Could you check a few things on this model? Use its own coordinates, in mm. Give positions to 0.01 mm unless a question says otherwise; leave off trailing zeros. Loops run counter-clockwise (first coordinate to the right, second up) from the corner with the lowest first, then second, coordinate; pieces in that order, holes last. Notation, with made-up numbers: M -34.5,-25.75 L -17.5,-25.75 A35 ccw -17.5,12.25 Z; hole C 4.25,-11 d11. An arc over 180 degrees is marked long. Use a Markdown table: item, result. Add a question column.
1) Suppose I cut it at B-B on y = -25.5. List the corners of the cut face in (x, z) for me, and give its area (3 significant figures).
2) Suppose I cut it at C-C on y = 26.5. List the corners of the cut face in (x, z) for me.
3) If I drill on line 1 along Y through (x, z) = (-42.5, 0.7); line 2 along X through (y, z) = (-60.5, 0.4); line 3 along X through (y, z) = (113, 0.55), over which ranges is the centre line in solid material (lowest first)? Write a range as [from, to].
4) Suppose I cut it at A-A on z = 1.05. Count the separate pieces of the cut face and the enclosed holes in it, and give its area (3 significant figures).
```python
from build123d import *

# Parameters (mm, degrees)
RESSALTO_EXTRUS_O1_DEPTH                     = 1.5
ESCAREADO_PARA_PARAFUSO_ALLEN_SEXTAV_2_COUNT = 2
ESCAREADO_PARA_PARAFUSO_ALLEN_SEXTAV_2_PITCH = 16.970294761
ESCAREADO_PARA_PARAFUSO_ALLEN_SEXTAV_3_COUNT = 2
ESCAREADO_PARA_PARAFUSO_ALLEN_SEXTAV_3_PITCH = 126.454837383
ESCAREADO_PARA_PARAFUSO_ALLEN_SEXTAV_4_COUNT = 2
ESCAREADO_PARA_PARAFUSO_ALLEN_SEXTAV_4_PITCH = 137.976919064
ESCAREADO_PARA_PARAFUSO_ALLEN_SEXTAV_5_COUNT = 2
ESCAREADO_PARA_PARAFUSO_ALLEN_SEXTAV_5_PITCH = 225.316554427
ESCAREADO_PARA_PARAFUSO_ALLEN_SEXTAV_6_COUNT = 2
ESCAREADO_PARA_PARAFUSO_ALLEN_SEXTAV_6_PITCH = 252.205372066
ESCAREADO_PARA_PARAFUSO_ALLEN_SEXTAV_7_COUNT = 2
ESCAREADO_PARA_PARAFUSO_ALLEN_SEXTAV_7_PITCH = 229.941146022
ESCAREADO_PARA_PARAFUSO_ALLEN_SEXTAV_8_COUNT = 2
ESCAREADO_PARA_PARAFUSO_ALLEN_SEXTAV_8_PITCH = 200.082309648


with BuildPart() as part:
    # Esboço1 → Ressalto-extrusão1 (new body)
    with BuildSketch(Plane.XY):
        Polygon((59.050720106, 130.399321825), (-58.939675618, 130.399321825), (-92.944477756, 89.873976712), (-92.944477756, 38.765530101), (-49.944477756, -12.47987438), (-49.944477756, -128.492963544), (-48.624354865, -129.600678175), (48.735399354, -129.600678175), (50.055522244, -128.492963544), (50.055522244, -12.47987438), (93.055522244, 38.765530101), (93.055522244, 89.873976712), align=None)
    extrude(amount=RESSALTO_EXTRUS_O1_DEPTH)

    # Esboço4 → Escareado para parafuso Allen sextavado escareado de M41 (revolve, cut)
    with BuildSketch(Plane(origin=(-63.227418691, 114.399321825, 1.5), x_dir=(0, -1, 0), z_dir=(1, 0, 0))):
        Polygon((0, 0), (0, 1.5), (2.25, 1.5), (2.25, 2.23), (4.48, 0), align=None)
    escareado_para_parafuso_allen_sextavado = revolve(axis=Axis((-63.227418691, 114.399321825, 7.85), (0, 0, -1)), mode=Mode.SUBTRACT)

    # Escareado para parafuso Allen sextav 2: Escareado para parafuso Allen sextavado escareado de M41 ×2
    with Locations(*[Vector(-0.64278761, -0.766044443, 0) * (i * ESCAREADO_PARA_PARAFUSO_ALLEN_SEXTAV_2_PITCH) for i in range(1, ESCAREADO_PARA_PARAFUSO_ALLEN_SEXTAV_2_COUNT)]):
        add(escareado_para_parafuso_allen_sextavado, mode=Mode.SUBTRACT)

    # Escareado para parafuso Allen sextav 3: Escareado para parafuso Allen sextavado escareado de M41 ×2
    with Locations(*[(i * ESCAREADO_PARA_PARAFUSO_ALLEN_SEXTAV_3_PITCH, 0, 0) for i in range(1, ESCAREADO_PARA_PARAFUSO_ALLEN_SEXTAV_3_COUNT)]):
        add(escareado_para_parafuso_allen_sextavado, mode=Mode.SUBTRACT)

    # Escareado para parafuso Allen sextav 4: Escareado para parafuso Allen sextavado escareado de M41 ×2
    with Locations(*[Vector(0.995551528, -0.094218657, 0) * (i * ESCAREADO_PARA_PARAFUSO_ALLEN_SEXTAV_4_PITCH) for i in range(1, ESCAREADO_PARA_PARAFUSO_ALLEN_SEXTAV_4_COUNT)]):
        add(escareado_para_parafuso_allen_sextavado, mode=Mode.SUBTRACT)

    # Escareado para parafuso Allen sextav 5: Escareado para parafuso Allen sextavado escareado de M41 ×2
    with Locations(*[Vector(0.468993043, -0.88320186, 0) * (i * ESCAREADO_PARA_PARAFUSO_ALLEN_SEXTAV_5_PITCH) for i in range(1, ESCAREADO_PARA_PARAFUSO_ALLEN_SEXTAV_5_COUNT)]):
        add(escareado_para_parafuso_allen_sextavado, mode=Mode.SUBTRACT)

    # Escareado para parafuso Allen sextav 6: Escareado para parafuso Allen sextavado escareado de M41 ×2
    with Locations(*[Vector(0.418991458, -0.907990175, 0) * (i * ESCAREADO_PARA_PARAFUSO_ALLEN_SEXTAV_6_PITCH) for i in range(1, ESCAREADO_PARA_PARAFUSO_ALLEN_SEXTAV_6_COUNT)]):
        add(escareado_para_parafuso_allen_sextavado, mode=Mode.SUBTRACT)

    # Escareado para parafuso Allen sextav 7: Escareado para parafuso Allen sextavado escareado de M41 ×2
    with Locations(*[Vector(0.090383741, -0.995907013, 0) * (i * ESCAREADO_PARA_PARAFUSO_ALLEN_SEXTAV_7_PITCH) for i in range(1, ESCAREADO_PARA_PARAFUSO_ALLEN_SEXTAV_7_COUNT)]):
        add(escareado_para_parafuso_allen_sextavado, mode=Mode.SUBTRACT)

    # Escareado para parafuso Allen sextav 8: Escareado para parafuso Allen sextavado escareado de M41 ×2
    with Locations(*[Vector(0.103871956, -0.994590678, 0) * (i * ESCAREADO_PARA_PARAFUSO_ALLEN_SEXTAV_8_PITCH) for i in range(1, ESCAREADO_PARA_PARAFUSO_ALLEN_SEXTAV_8_COUNT)]):
        add(escareado_para_parafuso_allen_sextavado, mode=Mode.SUBTRACT)


solid = part.part
```
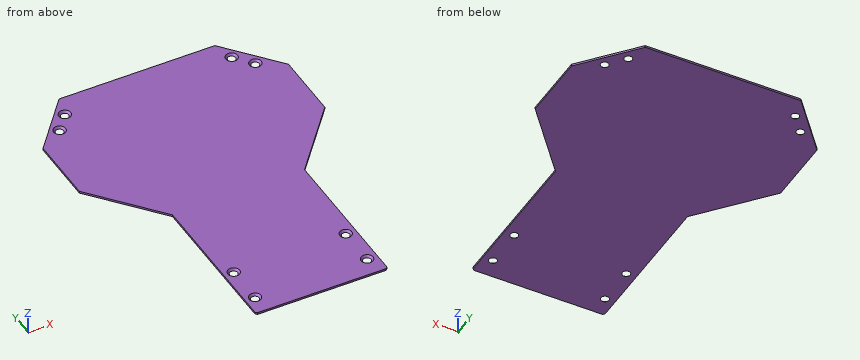
Answer block:
| question | item | result |
|---|---|---|
| 1 | outline | M -49.94,0 L 50.06,0 L 50.06,1.5 L -49.94,1.5 Z |
| 1 | area | 150 mm^2 |
| 2 | outline | M -82.65,0 L 82.76,0 L 82.76,1.5 L -82.65,1.5 Z |
| 3 | line 1 | y = [-129.6, -118.28], [-110.92, -88.28], [-80.92, 130.4] |
| 3 | line 2 | x = [-49.94, 50.06] |
| 3 | line 3 | x = [-73.54, -66.47], [-59.99, 59.99], [66.47, 73.65] |
| 4 | separate pieces | 1 |
| 4 | enclosed holes | 8 |
| 4 | area | 34,300 mm^2 |
